Input: part model. Units: mm. Frame: model coordinates. A direction names the side the tool comes from. Give positions to 0.01 mm unless a question says otherwise; leave off trailing zeros. Loops run counter-clockwise (first coordinate to the right, second up) from the corner with the lowest first, then second, coordinate; pieces in that order, holes last. Notation, with made-up numbers: M 68.5,-35 L 108.5,-35 A21 cw 108.5,-26 Z; hole C 39,34 d2. An arc over 180 degrees is marked long. Return JSON: item names as keys, results as strings. Group by question number.
```python
from build123d import *


with BuildPart() as f1:
    # F0 (on Front) → F1 (revolve)
    with BuildSketch(Plane.XZ):
        with BuildLine():
            Line((3.25, 2.5), (2.5, 2.5))
            ThreePointArc((2.5, 2.5), (1.767767, 4.267767), (0, 5))
            Line((0, 5), (0, -7))
            Line((0, -7), (0, -11))
            Line((0, -11), (3, -11))
            Line((3, -11), (3, -7))
            Line((3, -7), (4, -7))
            Line((4, -7), (4, 0))
            Line((4, 0), (4.75, 0))
            Line((4.75, 0), (4.75, 1))
            Line((4.75, 1), (3.25, 2.5))
        make_face()
    revolve(axis=Axis((0, 0, -3.678168), (0, 0, -1)))


solid = f1.part
```
Item 1: Section A-A, the plane z = -9. Return loops of the section in (x, y).
Item 2: First-contact query: pin 1 Ø2 at (x, z) = (3, -5) entering from +Y; pin 2 Ø1 at (y, z) = (1.5, -3.5) entering from +X; pin 3 Ø4 at (x, z) = (-1.5, -3.5) entering from -Y. Flat tips, straight axial feed; report the tip coordinate or a pass-through.
Item 3: Section B-B, the plane z = -2. Return loops of the section in (x, y), then the cut area to 3 significant figures.
Item 4: Material intervals for line 1 (Y direction, x = 0, z = -8); line 2 (Z direction, x = -1.75, y = 2.5); line 3 (Z direction, x = -2.75, y = 0.5), sorted ascending. Write a range as from..to.
Item 5: Reachability of faces 3 (the face through (2, 2, 2.5)), 4 (the face through (-1, -3, -7)), 5 (the face through (2.192, 4.214, 0.507)) from +Z, -Z, +X, -X, +Y, -Y: full face, straight path, thin tool, end or side. Return the list, or none.
Item 6: Pull-direction query (Y, two-part tool) for faces 1 (the face through (0, 0, -11)), 2 (the face through (-0.867, 3.905, -3.451)); classes: pulls with the +Y half, pulls with the -Y half, needs draft (parallel to the pull), parting line crosses it, or undercut.
Answer below:
{
 "1": {"outline": "C 0,0 d6"},
 "2": {"pin 1": "y = 3.46", "pin 2": "x = 3.87", "pin 3": "y = -4"},
 "3": {"outline": "C 0,0 d8", "area": "50.3 mm^2"},
 "4": {"line 1": "-3..3", "line 2": "-7..2.5", "line 3": "-11..2.5"},
 "5": {"face 3": "+Z", "face 4": "-Z", "face 5": "+Z, -Z"},
 "6": {"face 1": "needs draft", "face 2": "parting line crosses it"}
}
